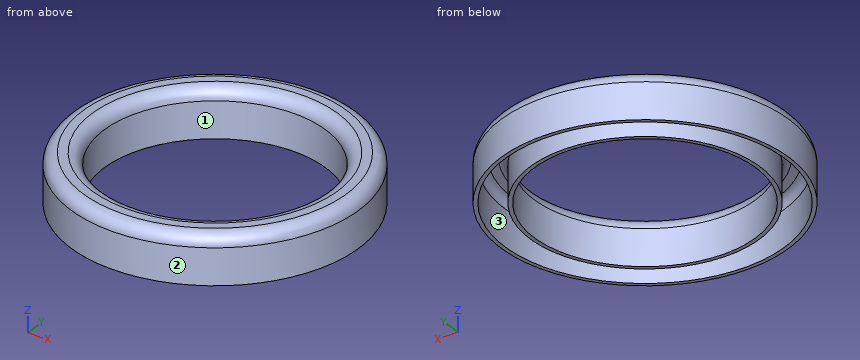
```python
from build123d import *

# Parameters (mm, degrees)
SKETCH1_R           = 35.73
SKETCH1_R_2         = 27.5
BOSS_EXTRUDE1_DEPTH = 12
FILLET1_R           = 3
SHELL1_T            = -1


with BuildPart() as part:
    # Sketch1 → Boss-Extrude1 (new body)
    with BuildSketch(Plane.XY):
        Circle(SKETCH1_R)
        Circle(SKETCH1_R_2, mode=Mode.SUBTRACT)
    extrude(amount=BOSS_EXTRUDE1_DEPTH)

    # Fillet1
    fillet1_edges = [part.edges().sort_by_distance(p)[0] for p in [
        (-35.73, 0, 12),
        (-27.5, 0, 12),
    ]]
    fillet(fillet1_edges, radius=FILLET1_R)

    # Shell1
    shell1_openings = [part.faces().sort_by_distance(p)[0] for p in [
        (-34.719402988, 0, 0),
    ]]
    offset(amount=SHELL1_T, openings=shell1_openings, kind=Kind.INTERSECTION)


solid = part.part
```
Build history of the part. All positions in model axes, mm. Face numbers are marked on the shaded views. Give positions to 0.01 mm unless a question says otherwise; leave off trailing zeros. Loops run counter-clockwise (first coordinate to the right, second up) from the corner with the lowest first, then second, coordinate; pieces in that order, holes last. Notation, with made-up numbers: (64.5, -15) - (87.5, -15) arc R20 ccw to (87.5, 24) - close; hole circle Ø6 at (78.25, -18). An arc over 180 degrees is marked (long way). Use a Markdown table: item, result.
(1) Band-saw the part on B-B (z = 4). Give the cut face in (x, y).
Taken from the geometry:
| item | result |
|---|---|
| outline | circle Ø71.46 at (0, 0); circle Ø57 at (0, 0); hole circle Ø69.46 at (0, 0); hole circle Ø55 at (0, 0) |
(2) Pull direction X, two halves, no side cores. Call the marked faces 1, 2 and 3: +X half, -X half, draft (parallel to the pull), parting line (faces both ways), or undercut.
Taken from the geometry:
| item | result |
|---|---|
| face 1 | undercut |
| face 2 | parting line |
| face 3 | undercut |
(3) Band-saw the part on A-A (y = 0). Give the cut face in (x, z).
Taken from the geometry:
| item | result |
|---|---|
| outline | (-35.73, 0) - (-34.73, 0) - (-34.73, 9) arc R2 cw to (-32.73, 11) - (-30.5, 11) arc R2 cw to (-28.5, 9) - (-28.5, 0) - (-27.5, 0) - (-27.5, 9) arc R3 ccw to (-30.5, 12) - (-32.73, 12) arc R3 ccw to (-35.73, 9) - close; (27.5, 0) - (28.5, 0) - (28.5, 9) arc R2 cw to (30.5, 11) - (32.73, 11) arc R2 cw to (34.73, 9) - (34.73, 0) - (35.73, 0) - (35.73, 9) arc R3 ccw to (32.73, 12) - (30.5, 12) arc R3 ccw to (27.5, 9) - close |
(4) Wall check: line 1 along Y through (x, z) = (0, 2); line 2 along X through (y, z) = (10, 4.25); line 3 along Y through (x, z) = (-23, 1.25). Give the ranges that are in metal, low to high.
Taken from the geometry:
| item | result |
|---|---|
| line 1 | -35.73 to -34.73, -28.5 to -27.5, 27.5 to 28.5, 34.73 to 35.73 |
| line 2 | -34.3 to -33.26, -26.69 to -25.62, 25.62 to 26.69, 33.26 to 34.3 |
| line 3 | -27.34 to -26.02, -16.83 to -15.07, 15.07 to 16.83, 26.02 to 27.34 |
(5) Drop flat-ended pins along their axis: pin 1 Ø5 at (x, z) = (-19.5, 3) entering from +Y; pin 2 Ø1 at (x, z) = (27, 10) entering from +Y. Give the stop position or say it passes through.
Taken from the geometry:
| item | result |
|---|---|
| pin 1 | y = 31.43 |
| pin 2 | y = 23.76 |
